from build123d import *

# Parameters (mm, degrees)
SKETCH1_R             = 73.025
BOSS_EXTRUDE1_DEPTH   = 6.35
CUT_EXTRUDE2_START    = -6.35
SKETCH2_R             = 3.175
CUT_EXTRUDE2_DEPTH    = 6.35
F_3_0MM_DOWEL_HOLE1_D = 3


with BuildPart() as part:
    # Sketch1 → Boss-Extrude1 (new body)
    with BuildSketch(Plane(origin=(0, 0, 0), x_dir=(1, 0, 0), z_dir=(0, 1, 0))):
        with Locations(Location((0, 0, 0), (0, 0, 270))):
            Circle(SKETCH1_R)
    extrude(amount=BOSS_EXTRUDE1_DEPTH)

    # Sketch2 → Cut-Extrude2 (cut)
    with BuildSketch(Plane(origin=(0, 6.35, 0), x_dir=(1, 0, 0), z_dir=(0, 1, 0)).offset(CUT_EXTRUDE2_START)):
        with BuildLine():
            ThreePointArc((61.150770614, -23.195291499), (0, -37.290063688), (-61.150770614, -23.195291499))
            ThreePointArc((-61.150770614, -23.195291499), (-66.917906968, -19.630921399), (-71.53671875, -14.667941079))
            ThreePointArc((-71.53671875, -14.667941079), (0, -73.025), (71.53671875, -14.667941079))
            ThreePointArc((71.53671875, -14.667941079), (66.917906968, -19.630921399), (61.150770614, -23.195291499))
        make_face()
        with BuildLine():
            ThreePointArc((-61.150770614, 23.195291499), (0, 37.290063688), (61.150770614, 23.195291499))
            ThreePointArc((61.150770614, 23.195291499), (66.917906968, 19.630921399), (71.53671875, 14.667941079))
            ThreePointArc((71.53671875, 14.667941079), (0, 73.025), (-71.53671875, 14.667941079))
            ThreePointArc((-71.53671875, 14.667941079), (-66.917906968, 19.630921399), (-61.150770614, 23.195291499))
        make_face()
        with Locations(Location((-50.8, 0, 0), (0, 0, 270))):
            Circle(SKETCH2_R)
        with Locations(Location((50.8, 0, 0), (0, 0, 270))):
            Circle(SKETCH2_R)
    extrude(amount=CUT_EXTRUDE2_DEPTH, mode=Mode.SUBTRACT)

    # Ø3.0mm Dowel Hole1 (through all)
    with Locations(Plane(origin=(0, 6.35, 0), x_dir=(1, 0, 0), z_dir=(0, 1, 0))):
        with Locations((-27.94, -15.24), (-2.54, -2.54)):
            Hole(F_3_0MM_DOWEL_HOLE1_D / 2)


solid = part.part
Can you work these out from the model? Positions are in its coordinate system, mm. Give positions to 0.01 mm unless a question says otherwise; leave off trailing zeros. Order: outer loops, then holes, each group sorted by start corner. A loop starts at its lowest first (then second) coordinate and runs counter-clockwise, first axis right, second up. Notation, with made-up numbers: M -10.75,66.25 L 27.25,66.25 A18 ccw 27.25,95.25 Z; hole C -26,40.25 d7. An arc over 180 degrees is marked long. Use one line per item in the form item = value. Start each with the question number.
Item 1: Will these pins go through, and if not, where does the flat tip stop? pin 1 Ø2 at (y, z) = (5.5, 17.5) entering from -X; pin 2 Ø2 at (x, y) = (-10, 0.5) entering from +Z; pin 3 Ø1 at (y, z) = (5.5, -15) entering from +X.
Item 2: If we section it at B-B (y = 1.25): Write out the boundary of the cut face in (x, z) (3 decimals).
Item 3: If I drill on line 1 along Z through (x, y) = (-2.54, 3.75); line 2 along Z through (x, y) = (-50.5, 1.5); line 3 along X through (y, z) = (5.25, 25.5), over which ranges is the centre line in solid material (lowest first)?
Item 4: If we section it at D-D (z = -13): Write out the boundary of the cut face in (x, y).
Item 5: We'd pull the mould along Z, two halves only. Please class faces 1 (the flat face through (1, 6.35, -1)), 2 (the cylindrical face through (-47.65, 3.13, -0.41)), 3 (the cylindrical face through (66.99, 3.13, 19.57)): +Z half, -Z half, draft (parallel to the pull), parting line (faces both ways), or undercut.
Item 6: If we section it at C-C (x = -27.94): Write out the boundary of the cut face in (y, z), then the cut area to 3 significant figures.
Item 7: If we section it at A-A (x = -2.54): Write out the boundary of the cut face in (y, z).
Outcome:
q1.pin_1 = -70.11
q1.pin_2 = 37
q1.pin_3 = 71.57
q2.outline = M -71.537,-14.668 A25.4 ccw -61.151,-23.195 A139.7 ccw 61.151,-23.195 A25.4 ccw 71.537,-14.668 A73.025 ccw 71.537,14.668 A25.4 ccw 61.151,23.195 A139.7 ccw -61.151,23.195 A25.4 ccw -71.537,14.668 A73.025 ccw Z; hole C -50.8,0 d6.35; hole C -27.94,15.24 d3; hole C -2.54,2.54 d3; hole C 50.8,0 d6.35
q3.line_1 = -37.27 to 1.04, 4.04 to 37.27
q3.line_2 = -27.84 to -3.16, 3.16 to 27.84
q3.line_3 = -56.17 to 56.17
q4.outline = M -71.86,0 L 71.86,0 L 71.86,6.35 L -71.86,6.35 Z
q5.face_1 = draft
q5.face_2 = undercut
q5.face_3 = +Z half
q6.outline = M 0,-34.47 L 6.35,-34.47 L 6.35,13.74 L 0,13.74 Z; M 0,16.74 L 6.35,16.74 L 6.35,34.47 L 0,34.47 Z
q6.area = 419 mm2
q7.outline = M 0,-37.27 L 6.35,-37.27 L 6.35,1.04 L 0,1.04 Z; M 0,4.04 L 6.35,4.04 L 6.35,37.27 L 0,37.27 Z
